The model under review builds one solid part; all positions refer to its coordinate system, in mm. Face numbers are marked on the shaded views. A direction names the side the tool comes from. Coordinates: 2 decimals unless noted, no trailing zeros. Order: outer loops, then holes, each group sorted by start corner. A loop starts at its lowest first (then second) coordinate and runs counter-clockwise, first axis right, second up. Notation, with made-up numbers: M 22,65.5 L 28,65.5 A28 cw 28,104.5 Z; hole C -38.75,46.25 d11. An arc over 180 degrees is marked long. One line per item, written item: value.
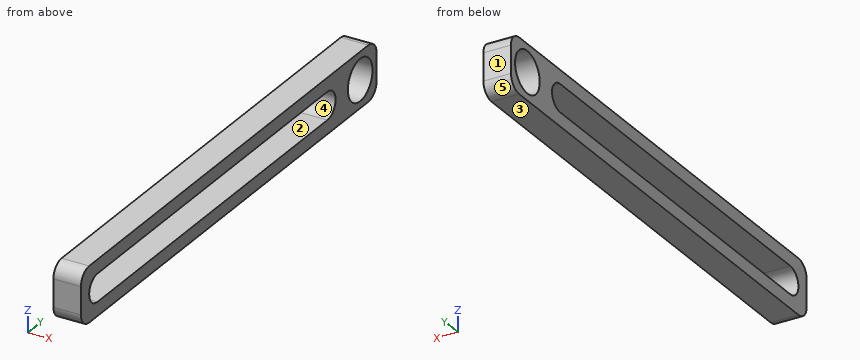
```python
from build123d import *

# Parameters (mm, degrees)
F0_R     = 9.525
F1_DEPTH = 6.35


with BuildPart() as f1:
    # F0 (on Right) → F1 (new body, symmetric)
    with BuildSketch(Plane.YZ):
        with BuildLine():
            ThreePointArc((114.3, 6.35), (112.440128, 10.840128), (107.95, 12.7))
            Line((107.95, 12.7), (-107.95, 12.7))
            ThreePointArc((-107.95, 12.7), (-112.440128, 10.840128), (-114.3, 6.35))
            Line((-114.3, 6.35), (-114.3, -6.35))
            ThreePointArc((-114.3, -6.35), (-112.440128, -10.840128), (-107.95, -12.7))
            Line((-107.95, -12.7), (107.95, -12.7))
            ThreePointArc((107.95, -12.7), (112.440128, -10.840128), (114.3, -6.35))
            Line((114.3, -6.35), (114.3, 6.35))
        make_face()
        with BuildLine():
            ThreePointArc((-101.6, -6.35), (-107.95, 0), (-101.6, 6.35))
            Line((-101.6, 6.35), (76.2, 6.35))
            ThreePointArc((76.2, 6.35), (82.55, 0), (76.2, -6.35))
            Line((76.2, -6.35), (-101.6, -6.35))
        make_face(mode=Mode.SUBTRACT)
        with Locations((101.6, 0)):
            Circle(F0_R, mode=Mode.SUBTRACT)
    extrude(amount=F1_DEPTH, both=True)


solid = f1.part
```
(1) We need section A-A, the plane z = 0. State the section outline as (x, y) points (3 decimals), plus the area to 3 significant figures.
Geometry results:
outline: M -6.35,-114.3 L 6.35,-114.3 L 6.35,-107.95 L -6.35,-107.95 Z; M -6.35,82.55 L 6.35,82.55 L 6.35,92.075 L -6.35,92.075 Z; M -6.35,111.125 L 6.35,111.125 L 6.35,114.3 L -6.35,114.3 Z
area: 242 mm2
(2) Mouldability with a two-part tool opening along Y and no side actions: class the marked faces 3, 4 and 5 as +Y half, -Y half, draft (parallel to the pull), parting line (faces both ways), or undercut.
Geometry results:
face 3: draft
face 4: undercut
face 5: +Y half
(3) For L1, parallel to Y at x = 3.25, z = -3.75; L2, parallel to Z at x = 1.5, y = 57; L3, parallel to Y at x = 1.5, z = 3.5, list the stretches that pass through material, from the lowest coordinate up.
Geometry results:
L1: y = -114.3 to -106.72, 81.32 to 92.84, 110.36 to 114.3
L2: z = -12.7 to -6.35, 6.35 to 12.7
L3: y = -114.3 to -106.9, 81.5 to 92.74, 110.46 to 114.3
(4) Tool access review of the marked faces 1 and 2: name each direction out of +Z, -Z, +X, -X, +Y, -Y from which nothing blocks a thin tool from reaching the whole face with its end or side.
Geometry results:
face 1: +Z, -Z, +X, -X, +Y
face 2: +X, -X
(5) We need section C-C, the plane x = 3. State the section outline as (y, z) points (3 decimals), plus the area to 3 significant figures.
Geometry results:
outline: M -114.3,-6.35 A6.35 ccw -107.95,-12.7 L 107.95,-12.7 A6.35 ccw 114.3,-6.35 L 114.3,6.35 A6.35 ccw 107.95,12.7 L -107.95,12.7 A6.35 ccw -114.3,6.35 Z; hole M -101.6,-6.35 L 76.2,-6.35 A6.35 ccw 76.2,6.35 L -101.6,6.35 A6.35 ccw Z; hole C 101.6,0 d19.05
area: 3,100 mm2
(6) We need section B-B, the plane y = 32.5. State the section outline as (x, z) points, plus the area to 3 significant figures.
Geometry results:
outline: M -6.35,-12.7 L 6.35,-12.7 L 6.35,-6.35 L -6.35,-6.35 Z; M -6.35,6.35 L 6.35,6.35 L 6.35,12.7 L -6.35,12.7 Z
area: 161 mm2
